Check sheet for the drawn part. Datum: minimum x, y, z corner. Units: mm. A direction names the side the tool comes from. Give positions to 0.01 mm unless a question says otherwise; leave off trailing zeros. Loops run counter-clockwise (first coordinate to the right, second up) from the corner with the lowest first, then second, coordinate; pieces in that order, holes last. Notation, with made-up numbers: (25, -23) - (54, -23) arc R20 ccw to (54, -2) - close; hole circle Ø11 at (-32.5, 63.25). An arc over 180 degrees is marked (long way). One line per item, written item: value. Start each with the question number.
1. Sectioned sample at C-C (y = 175). Record the cut outline in (x, z).
2. Sectioned sample at D-D (y = 234). Record the cut outline in (x, z), plus the area to 3 significant figures.
3. Sectioned sample at B-B (z = 14). Record the cut outline in (x, y).
4. Access from +Z, -Z, +X, -X, +Y, -Y to the whole of each face (thin tool, end or side, straight path). Record for the marked faces 4 and 5.
5. Sectioned sample at A-A (x = 53.5). Record the cut outline in (y, z), plus the area to 3 significant figures.
6. Gauge pin test, flat end, axial feed: pin 1 (10 mm diameter, centred on x = 19, z = 50, fed in from -Y). Record the tip position at first contact, or that the pin passes through.
7. Scan lines: L1, parallel to X at y = 144.5, z = 9; L2, parallel to Z at x = 19, y = 221. Record each from-to range of solid material in increasing order. Write a range as [from, to].
8. Mould release check, pull along Z, two halves, no side actions. Record for the marked faces 1, 2 and 3: pulls with the +Z half, pulls with the -Z half, needs draft (parallel to the pull), parting line crosses it, or undercut.
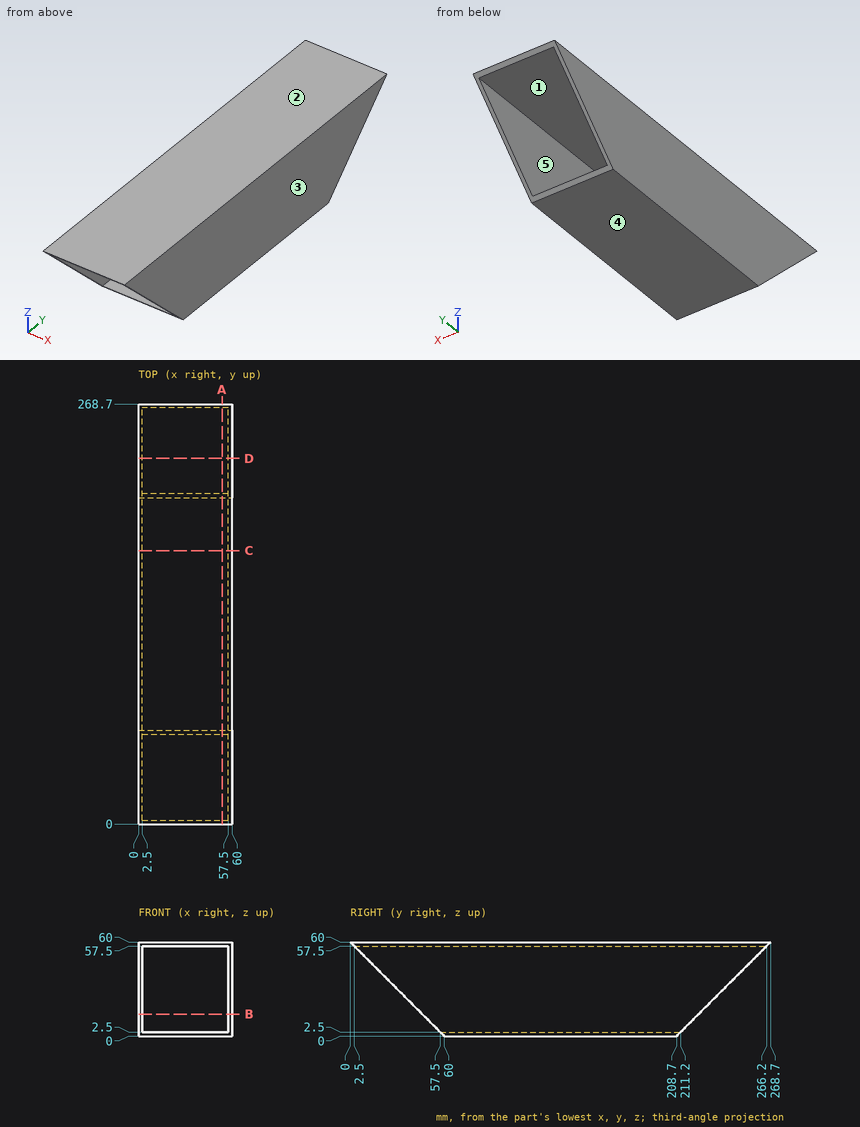
Results are:
1. outline: (0, 0) - (60, 0) - (60, 60) - (0, 60) - close; hole (2.5, 2.5) - (57.5, 2.5) - (57.5, 57.5) - (2.5, 57.5) - close
2. outline: (0, 25.3) - (2.5, 25.3) - (2.5, 57.5) - (57.5, 57.5) - (57.5, 25.3) - (60, 25.3) - (60, 60) - (0, 60) - close
2. area: 311 mm^2
3. outline: (0, 46) - (2.5, 46) - (2.5, 222.7) - (0, 222.7) - close; (57.5, 46) - (60, 46) - (60, 222.7) - (57.5, 222.7) - close
4. face 4: -Z, +X, -X, +Y, -Y
4. face 5: +Y, -Y
5. outline: (0, 60) - (2.5, 57.5) - (266.2, 57.5) - (268.7, 60) - close; (57.5, 2.5) - (60, 0) - (208.7, 0) - (211.2, 2.5) - close
5. area: 1,040 mm^2
6. pin 1: passes through
7. L1: x = [0, 2.5], [57.5, 60]
7. L2: z = [57.5, 60]
8. face 1: undercut
8. face 2: pulls with the +Z half
8. face 3: needs draft
